from build123d import *

# Parameters (mm, degrees)
F0_R     = 22.5
F1_DEPTH = 20


with BuildPart() as f1:
    # F0 (on Front) → F1 (new body)
    with BuildSketch(Plane.XZ):
        Polygon((16.897677, 50), (-16.897677, 50), (-50, 30.941529), (-50, -30.941529), (-16.897677, -50), (16.897677, -50), (50, -30.941529), (50, 30.941529), align=None)
        Circle(F0_R, mode=Mode.SUBTRACT)
        Polygon((-50, -30.941529), (-50, 30.941529), (-65.928897, 0), align=None)
        Polygon((65.928897, 0), (50, 30.941529), (50, -30.941529), align=None)
    extrude(amount=F1_DEPTH)


solid = f1.part
Verification items for the finished model (mm, model axes). Give positions to 0.01 mm unless a question says otherwise; leave off trailing zeros. Loops run counter-clockwise (first coordinate to the right, second up) from the corner with the lowest first, then second, coordinate; pieces in that order, holes last.
1. Material ranges on probe 1 along Z at (x, y) = (0, -14.5); probe 2 along Z at (x, y) = (-8, -5.25); probe 3 along Z at (x, y) = (-27, -1.25), recorded low to high.
Derived:
probe 1: z = -50 to -22.5, 22.5 to 50
probe 2: z = -50 to -21.03, 21.03 to 50
probe 3: z = -44.18 to 44.18
2. Cross-section at D-D on x = -58. Record the cut outline in (y, z).
Derived:
outline: (-20, -15.4) - (0, -15.4) - (0, 15.4) - (-20, 15.4) - close
3. Cross-section at A-A on x = 0. Record the cut outline in (y, z).
Derived:
outline: (-20, -50) - (0, -50) - (0, -22.5) - (-20, -22.5) - close; (-20, 22.5) - (0, 22.5) - (0, 50) - (-20, 50) - close
4. Go/stop test with flat-tipped pins: P1, Ø12, axis at x = -34, y = -18, coming from the -Z side; P2, Ø1, axis at y = -2.5, z = 25.5, coming from the +X side; P3, Ø8, axis at y = -11, z = 24.5, coming from the +X side. Record where each tip stops, or that it passes through.
Derived:
P1: stops at z = -43.61
P2: stops at x = 53.06
P3: stops at x = 55.38
5. Release check for a two-part mould opening along X. For faces 1 (the cylindrical face through (10.382, -9.86, -19.961)), 2 (the flat face through (58.08, -9.86, 15.25)), 3 (the flat face through (0, -10, 50)) record: +X half, -X half, draft (parallel to the pull), parting line (faces both ways), or undercut.
Derived:
face 1: undercut
face 2: +X half
face 3: draft
6. Cross-section at B-B on y = -14.5. Record the cut outline in (x, z), and give its area (3 significant figures).
Derived:
outline: (-65.93, 0) - (-50, -30.94) - (-16.9, -50) - (16.9, -50) - (50, -30.94) - (65.93, 0) - (50, 30.94) - (16.9, 50) - (-16.9, 50) - (-50, 30.94) - close; hole circle Ø45 at (0, 0)
area: 8,130 mm2
7. Cross-section at C-C on z = -9.5. Record the cut outline in (x, y).
Derived:
outline: (-61.04, -20) - (-20.4, -20) - (-20.4, 0) - (-61.04, 0) - close; (20.4, -20) - (61.04, -20) - (61.04, 0) - (20.4, 0) - close
